Part print with two shaded views. Sizes in mm from the minimum x, y, z corner. A direction names the side the tool comes from. Round coordinates to 2 decimals unless told otherwise and drop trailing zeros. Loops run counter-clockwise (first coordinate to the right, second up) from the corner with the lowest first, then second, coordinate; pieces in that order, holes last. Notation, with made-up numbers: (80.5, -29) -> (110.5, -29) arc R13 ccw to (110.5, -8) -> close; hole circle Ø10 at (-34, 49). An arc over 180 degrees is marked (long way). Use a Markdown table: item, result. Add a question column.
Item 1: Probe line 1 (Z direction, x = 35, y = 7); line 2 (Y direction, x = 50, z = 89.5) (1 decimal); line 3 (Z direction, x = 38, y = 63.5). List the from-to ranges inside material, lowest first. Write a range as [from, to].
Item 2: Which spindle directions (+Z, -Z, +X, -X, +Y, -Y) get a long thin tool onto all of the face, cutting with end or side? Do the marked faces 1 and 2. Say none if no direction does.
Item 3: Flat gauge pins, fed straight in: pin 1 (17 mm diameter, centred on x = 35, z = 71.52, fed in from +Y) (1 decimal); pin 2 (12 mm diameter, centred on x = 35.5, y = 23.5, fed in from -Z); pin 3 (8 mm diameter, centred on x = 20.5, y = 40, fed in from +Z). Where does each tip first touch, or does it go through?
Item 4: Cut at A-A, the plane x = 35. List the corners of the cut face in (y, z) (1 decimal), plus the area to 3 significant figures.
Item 5: Two-plate mould, pull along Z, no slides. Class the marked faces 3, 4 and 5: pulls with the +Z half, pulls with the -Z half, needs draft (parallel to the pull), parting line crosses it, or undercut.
Item 6: Cut at C-C, the plane x = 13. List the corners of the cut face in (y, z) (1 decimal), plus the area to 3 significant figures.
Item 7: Cut at B-B, the plane z = 76.5. List the corners of the cut face in (x, y) (1 decimal), plus the area to 3 significant figures.
Item 8: Cut at D-D, the plane z = 49. List the corners of the cut face in (x, y) (1 decimal), plus the area to 3 significant figures.
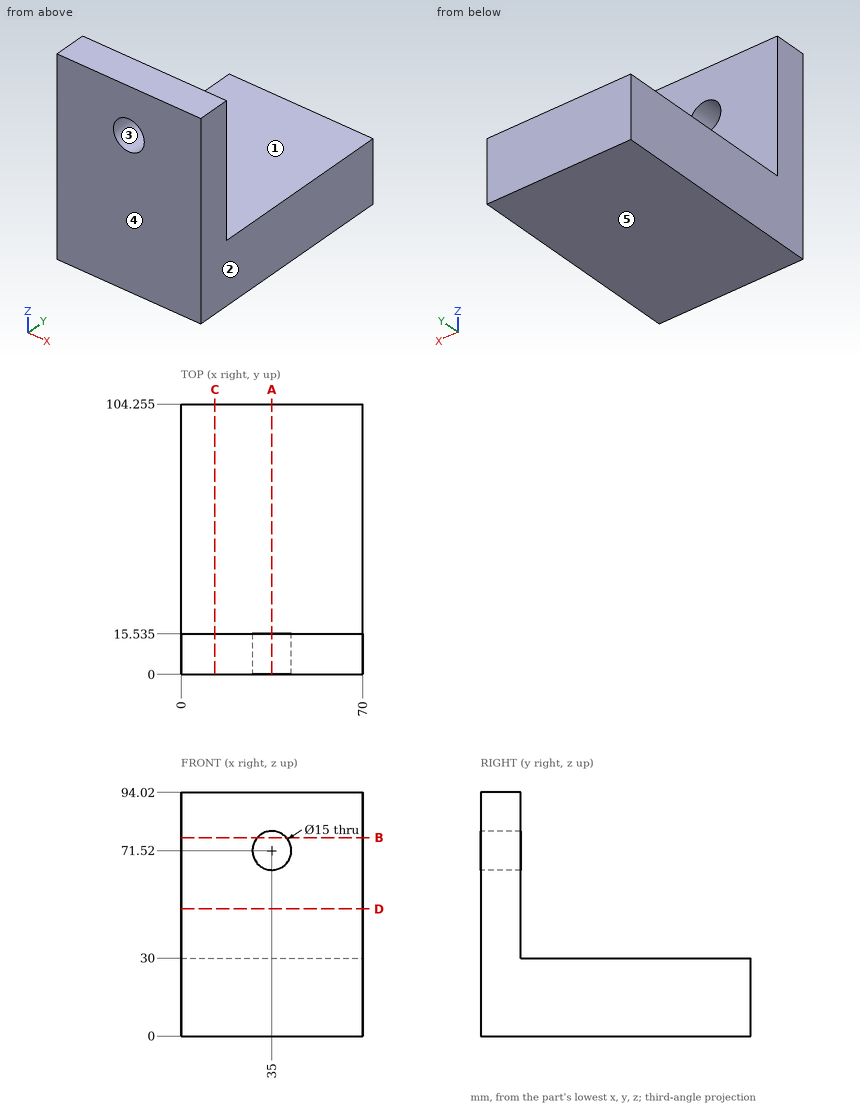
A:
| question | item | result |
|---|---|---|
| 1 | line 1 | z = [0, 64.02], [79.02, 94.02] |
| 1 | line 2 | y = [0, 15.5] |
| 1 | line 3 | z = [0, 30] |
| 2 | face 1 | +Z, +X, -X, +Y |
| 2 | face 2 | +Z, -Z, +X, +Y, -Y |
| 3 | pin 1 | stops at y = 15.5 |
| 3 | pin 2 | stops at z = 0 |
| 3 | pin 3 | stops at z = 30 |
| 4 | outline | (0, 0) -> (104.3, 0) -> (104.3, 30) -> (15.5, 30) -> (15.5, 64) -> (0, 64) -> close; (0, 79) -> (15.5, 79) -> (15.5, 94) -> (0, 94) -> close |
| 4 | area | 3,890 mm^2 |
| 5 | face 3 | undercut |
| 5 | face 4 | needs draft |
| 5 | face 5 | pulls with the -Z half |
| 6 | outline | (0, 0) -> (104.3, 0) -> (104.3, 30) -> (15.5, 30) -> (15.5, 94) -> (0, 94) -> close |
| 6 | area | 4,120 mm^2 |
| 7 | outline | (0, 0) -> (29.4, 0) -> (29.4, 15.5) -> (0, 15.5) -> close; (40.6, 0) -> (70, 0) -> (70, 15.5) -> (40.6, 15.5) -> close |
| 7 | area | 913 mm^2 |
| 8 | outline | (0, 0) -> (70, 0) -> (70, 15.5) -> (0, 15.5) -> close |
| 8 | area | 1,090 mm^2 |
